```python
from build123d import *

# Parameters (mm, degrees)
BOSS_EXTRUDE1_DEPTH      = 5
BOSS_EXTRUDE1_DEPTH_BACK = 5
SKETCH1_R                = 28.575
CUT_EXTRUDE12_START      = 29
SKETCH15_R               = 2
CUT_EXTRUDE12_DEPTH      = 5
CUT_EXTRUDE13_START      = -29
SKETCH16_R               = 2
CUT_EXTRUDE13_DEPTH      = 5
CUT_EXTRUDE14_START      = -15
CUT_EXTRUDE14_DEPTH      = 2.9
CUT_EXTRUDE15_DEPTH      = 41.719298415
CUT_EXTRUDE15_DEPTH_BACK = 41.719298415
SKETCH21_W               = 7
SKETCH21_H               = 2.9
CUT_EXTRUDE16_DEPTH      = 5
SKETCH22_R               = 2
CUT_EXTRUDE17_DEPTH      = 55.785547976


with BuildPart() as part:
    # Sketch1 → Boss-Extrude1 (new, two sides: drawn at the far end of the back side and taken through both)
    with BuildSketch(Plane.XY.offset(-BOSS_EXTRUDE1_DEPTH_BACK)):
        Circle(SKETCH1_R)
    extrude(amount=BOSS_EXTRUDE1_DEPTH + BOSS_EXTRUDE1_DEPTH_BACK)

    # Sketch15 → Cut-Extrude12 (cut)
    with BuildSketch(Plane(origin=(0, 0, 0), x_dir=(1, 0, 0), z_dir=(0, 1, 0)).offset(CUT_EXTRUDE12_START)):
        with Locations(Location((0, 0, 0), (0, 0, 270))):
            Circle(SKETCH15_R)
    extrude(amount=-CUT_EXTRUDE12_DEPTH, mode=Mode.SUBTRACT)

    # Sketch16 → Cut-Extrude13 (cut)
    with BuildSketch(Plane(origin=(0, 0, 0), x_dir=(0, 0, -1), z_dir=(1, 0, 0)).offset(CUT_EXTRUDE13_START)):
        with Locations(Location((0, 0, 0), (0, 0, 180))):
            Circle(SKETCH16_R)
    cut_extrude13 = extrude(amount=CUT_EXTRUDE13_DEPTH, mode=Mode.SUBTRACT)

    # Sketch19 → Cut-Extrude14 (cut)
    with BuildSketch(Plane(origin=(0, 0, 0), x_dir=(1, 0, 0), z_dir=(0, 1, 0)).offset(CUT_EXTRUDE14_START)):
        Polygon((0, 4.041451884), (-3.5, 2.020725942), (-3.5, -2.020725942), (0, -4.041451884), (3.5, -2.020725942), (3.5, 2.020725942), align=None)
    extrude(amount=-CUT_EXTRUDE14_DEPTH, mode=Mode.SUBTRACT)

    # Sketch20 → Cut-Extrude15 (cut, two sides: drawn at the far end of the back side and taken through both)
    with BuildSketch(Plane.XY.offset(-CUT_EXTRUDE15_DEPTH_BACK)):
        with BuildLine():
            Line((-22.5, 0), (22.5, 0))
            ThreePointArc((22.5, 0), (0, 22.5), (-22.5, 0))
        make_face()
    extrude(amount=CUT_EXTRUDE15_DEPTH + CUT_EXTRUDE15_DEPTH_BACK, mode=Mode.SUBTRACT)

    # Mirror1: Cut-Extrude13 across plane
    add(cut_extrude13.mirror(Plane(origin=(0, 0, 0), x_dir=(0, 0, 1), z_dir=(1, 0, 0))), mode=Mode.SUBTRACT)

    # Sketch21 → Cut-Extrude16 (cut)
    with BuildSketch(Plane.XY.offset(5)):
        with Locations((0, -16.45)):
            Rectangle(SKETCH21_W, SKETCH21_H)
    extrude(amount=-CUT_EXTRUDE16_DEPTH, mode=Mode.SUBTRACT)

    # Sketch22 → Cut-Extrude17 (cut, through all)
    with BuildSketch(Plane(origin=(0, -17.9, 0), x_dir=(1, 0, 0), z_dir=(0, 1, 0))):
        with Locations(Location((0, 0, 0), (0, 0, 270))):
            Circle(SKETCH22_R)
    extrude(amount=-CUT_EXTRUDE17_DEPTH, mode=Mode.SUBTRACT)


solid = part.part
```
Read the model definition and answer for the solid it produces. Units are mm, in the model's axes. A direction names the side the tool comes from. Give positions to 0.01 mm unless a question says otherwise; leave off trailing zeros. Write each loop counter-clockwise with the first axis right and the second up, starting at its lowest first coordinate (ties: lowest second). Pieces come first, ordered by that corner, then holes. Notation, with made-up numbers: (-30.5, 79) - (17.5, 79) arc R26 ccw to (17.5, 95) - close; hole circle Ø10 at (-39.75, 24). An arc over 180 degrees is marked (long way). Write item = value, one per line. Start each with the question number.
Item 1: Find section A-A (y = 12.5). Give the vertices of the cut face in (x, z).
Item 2: Find section D-D (z = 0). Give the vertices of the cut face in (x, y) (3 decimals), then the cut area to 3 significant figures.
Item 3: Find section B-B (x = 8.5). Give the vertices of the cut face in (y, z).
Item 4: A tool of negligible diameter and unlimited length cuts with its end or side. For faces 5 (the cylindrical face through (-2, -23, 0)), 6 (the flat face through (3.5, -16, 2)), 7 (the flat face through (0, 24, 0)), from which of +Z, -Z, +X, -X, +Y, -Y can it reach the whole face along a straight path? Write none if from no direction.
Item 5: Each of these flat-tipped pins is pushed along its axis until it touches: P1, Ø2, axis at y = 0, z = 0.5, coming from the -X side; P2, Ø3, axis at x = 0, z = 0, coming from the +Y side; P3, Ø2, axis at x = 0.5, z = -0.5, coming from the -Y side; P4, Ø3, axis at x = 0, z = 1, coming from the +Y side (3 decimals). Where does it stop, or does it pass through?
Item 6: Find section C-C (z = 3). Give the vertices of the cut face in (x, y) (3 decimals), then the cut area to 3 significant figures.
Item 7: The mould has two halves that part along X. Classify faces 1 (the flat face through (24, 0, 0)), 2 (the cylindrical face through (-26.32, -0.601, 1.908)), 3 (the cylindrical face through (27.255, 8.583, -0.07)), 4 (the flat face through (-3.5, -16, 2)): +X half, -X half, draft (parallel to the pull), parting line (faces both ways), or undercut.
Item 8: Find the intervals of material crossed by probe 1 along X at (y, z) = (-23.5, 0); probe 2 along Z at (x, y) = (0, -22.5); probe 3 along X at (y, z) = (-19.75, 0), in increasing order. Write a range as [from, to].
Response:
q1.outline = (-25.7, -5) - (-18.71, -5) - (-18.71, 5) - (-25.7, 5) - close; (18.71, -5) - (25.7, -5) - (25.7, 5) - (18.71, 5) - close
q2.outline = (-28.505, -2) arc R28.575 ccw to (-2, -28.505) - (-2, -17.9) - (-3.5, -17.9) - (-3.5, -15) - (3.5, -15) - (3.5, -17.9) - (2, -17.9) - (2, -28.505) arc R28.575 ccw to (28.505, -2) - (24, -2) - (24, 2) - (28.505, 2) arc R28.575 ccw to (2, 28.505) - (2, 24) - (-2, 24) - (-2, 28.505) arc R28.575 ccw to (-28.505, 2) - (-24, 2) - (-24, -2) - close; hole (-22.5, 0) - (22.5, 0) arc R22.5 ccw to start
q2.area = 1,650 mm²
q3.outline = (-27.28, -5) - (0, -5) - (0, 5) - (-27.28, 5) - close; (20.83, -5) - (27.28, -5) - (27.28, 5) - (20.83, 5) - close
q4.face_5 = -Y
q4.face_6 = +Z
q4.face_7 = +Y
q5.P1 = -24
q5.P2 = 24
q5.P3 = -15
q5.P4 = 28.575
q6.outline = circle Ø57.15 at (0, 0); hole (-22.5, 0) - (22.5, 0) arc R22.5 ccw to start; hole (-3.5, -17.9) - (3.5, -17.9) - (3.5, -15) - (-3.5, -15) - close
q6.area = 1,750 mm²
q7.face_1 = +X half
q7.face_2 = draft
q7.face_3 = parting line
q7.face_4 = undercut
q8.probe_1 = [-16.26, -2], [2, 16.26]
q8.probe_2 = [-5, -2], [2, 5]
q8.probe_3 = [-20.65, -2], [2, 20.65]
